Part model, mm, in its own coordinate system. Face numbers are marked on the shaded views. A direction names the side the tool comes from. Give positions to 0.01 mm unless a question says otherwise; leave off trailing zeros. Write each loop counter-clockwise with the first axis right and the second up, starting at its lowest first coordinate (ties: lowest second). Pieces come first, ordered by that corner, then holes. Notation, with made-up numbers: (-33, 85) - (-20, 85) arc R28 cw to (-20, 104) - close; hole circle Ø9 at (34, -39.75). An arc over 180 degrees is marked (long way). Answer as a JSON object with one key per item and string values. Group by question number.
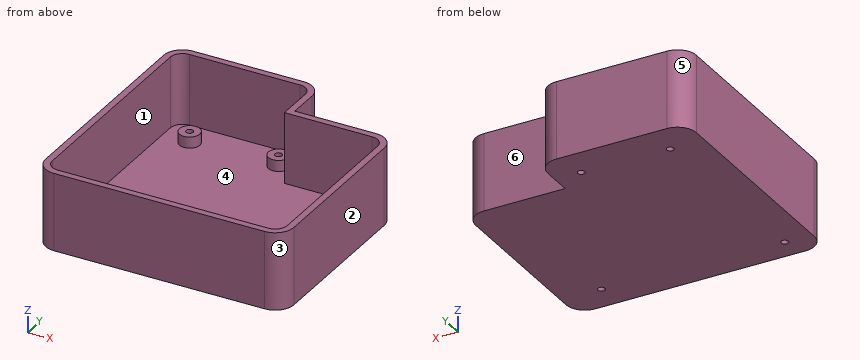
```python
from build123d import *

# Parameters (mm, degrees)
SKETCH1_R           = 1.6
BOSS_EXTRUDE1_DEPTH = 35
SHELL3_T            = -3
CUT_EXTRUDE2_DEPTH  = 27


with BuildPart() as part:
    # Sketch1 → Boss-Extrude1 (new body)
    with BuildSketch(Plane.XY):
        with BuildLine():
            Line((41.47958643, 169.703196001), (-8.43041357, 169.703196001))
            ThreePointArc((-8.43041357, 169.703196001), (-14.44082121, 167.213603641), (-16.93041357, 161.203196001))
            Line((-16.93041357, 161.203196001), (-16.93041357, 66.203196001))
            ThreePointArc((-16.93041357, 66.203196001), (-14.44082121, 60.192788361), (-8.43041357, 57.703196001))
            Line((-8.43041357, 57.703196001), (86.56958643, 57.703196001))
            ThreePointArc((86.56958643, 57.703196001), (92.57999407, 60.192788361), (95.06958643, 66.203196001))
            Line((95.06958643, 66.203196001), (95.06958643, 138.923196001))
            ThreePointArc((95.06958643, 138.923196001), (92.57999407, 144.933603641), (86.56958643, 147.423196001))
            Line((86.56958643, 147.423196001), (84.57958643, 147.423196001))
            Line((84.57958643, 147.423196001), (78.22958643, 147.423196001))
            Line((78.22958643, 147.423196001), (56.63958643, 147.423196001))
            Line((56.63958643, 147.423196001), (50.28958643, 147.423196001))
            Line((50.28958643, 147.423196001), (49.947630422, 147.423196001))
            Line((49.947630422, 147.423196001), (49.97958643, 161.203196001))
            ThreePointArc((49.97958643, 161.203196001), (47.48999407, 167.213603641), (41.47958643, 169.703196001))
        make_face()
        with Locations((-1.583516975, 154.760976138)):
            Circle(SKETCH1_R, mode=Mode.SUBTRACT)
        with Locations((38.108590224, 155.552573365)):
            Circle(SKETCH1_R, mode=Mode.SUBTRACT)
        with Locations((-4.549842033, 67.784537285)):
            Circle(SKETCH1_R, mode=Mode.SUBTRACT)
        with Locations((76.81802316, 70.207451643)):
            Circle(SKETCH1_R, mode=Mode.SUBTRACT)
    extrude(amount=BOSS_EXTRUDE1_DEPTH)

    # Shell3
    shell3_openings = [part.faces().sort_by_distance(p)[0] for p in [
        (36.150005596, 109.720855489, 35),
    ]]
    offset(amount=SHELL3_T, openings=shell3_openings, kind=Kind.INTERSECTION)

    # Sketch4 → Cut-Extrude2 (cut)
    with BuildSketch(Plane.XY.offset(35)):
        with BuildLine():
            Line((41.47958643, 164.703196001), (-8.43041357, 164.703196001))
            ThreePointArc((-8.43041357, 164.703196001), (-10.905287304, 163.678069735), (-11.93041357, 161.203196001))
            Line((-11.93041357, 161.203196001), (-11.93041357, 66.203196001))
            ThreePointArc((-11.93041357, 66.203196001), (-10.905287304, 63.728322267), (-8.43041357, 62.703196001))
            Line((-8.43041357, 62.703196001), (86.56958643, 62.703196001))
            ThreePointArc((86.56958643, 62.703196001), (89.044460164, 63.728322267), (90.06958643, 66.203196001))
            Line((90.06958643, 66.203196001), (90.06958643, 138.923196001))
            ThreePointArc((90.06958643, 138.923196001), (89.044460164, 141.398069735), (86.56958643, 142.423196001))
            Line((86.56958643, 142.423196001), (44.936021909, 142.423196001))
            Line((44.936021909, 142.423196001), (44.979583495, 161.207728174))
            ThreePointArc((44.979583495, 161.207728174), (43.95285728, 163.679671582), (41.47958643, 164.703196001))
        make_face()
    extrude(amount=-CUT_EXTRUDE2_DEPTH, mode=Mode.SUBTRACT)


solid = part.part
```
1) Saw through at D-D (x = 1.5). List the corners of the cut face in (y, z), and give its area (3 significant figures).
2) Saw through at A-A (z = 28). List the corners of the cut face in (x, y), and give its area (3 significant figures).
3) Two-plate mould, pull along Y, no slides. Class the marked faces 1, 2 and 3: +Y half, -Y half, draft (parallel to the pull), parting line (faces both ways), or undercut.
4) Drill centre lines: line 1 along X through (y, z) = (95.5, 17); line 2 along Y through (x, z) = (27.5, 14.5); line 3 along X through (y, z) = (161.5, 7). Where is each one in solid material? Low to high. Write a range as from..to.
5) Drop flat-ended pins along their axis: P1, Ø10, axis at x = -2, y = 156, coming from the +Z side; P2, Ø1.9, axis at x = -1.58, y = 154.76, coming from the +Z side; P3, Ø10.5, axis at x = 60.5, z = 23, coming from the +Y side. Give the stop position or say it passes through.
6) Saw through at C-C (x = 13). List the corners of the cut face in (y, z), and give its area (3 significant figures).
7) Which spindle directions (+Z, -Z, +X, -X, +Y, -Y) get a long thin tool onto all of the face, cutting with end or side? Do the marked faces 4, 5 and 6. Say none if no direction does.
8) Saw through at B-B (y = 81.5). List the corners of the cut face in (x, z), and give its area (3 significant figures).
Checks:
{
 "1": {"outline": "(57.7, 0) - (169.7, 0) - (169.7, 35) - (166.7, 35) - (166.7, 3) - (158.17, 3) - (158.17, 8) - (151.35, 8) - (151.35, 3) - (60.7, 3) - (60.7, 35) - (57.7, 35) - close", "area": "562 mm2"},
 "2": {"outline": "(-16.93, 66.2) arc R8.5 ccw to (-8.43, 57.7) - (86.57, 57.7) arc R8.5 ccw to (95.07, 66.2) - (95.07, 138.92) arc R8.5 ccw to (86.57, 147.42) - (49.95, 147.42) - (49.98, 161.2) arc R8.5 ccw to (41.48, 169.7) - (-8.43, 169.7) arc R8.5 ccw to (-16.93, 161.2) - close; hole (-13.93, 66.2) arc R5.5 ccw to (-8.43, 60.7) - (86.57, 60.7) arc R5.5 ccw to (92.07, 66.2) - (92.07, 138.92) arc R5.5 ccw to (86.57, 144.42) - (46.94, 144.42) - (46.98, 161.21) arc R5.5 ccw to (41.48, 166.7) - (-8.43, 166.7) arc R5.5 ccw to (-13.93, 161.2) - close", "area": "1,260 mm2"},
 "3": {"face 1": "undercut", "face 2": "draft", "face 3": "-Y half"},
 "4": {"line 1": "-16.93..-13.93, 92.07..95.07", "line 2": "57.7..60.7, 166.7..169.7", "line 3": "-16.93..-13.92, 46.97..49.97"},
 "5": {"P1": "z = 8", "P2": "through", "P3": "y = 147.42"},
 "6": {"outline": "(57.7, 0) - (169.7, 0) - (169.7, 35) - (166.7, 35) - (166.7, 3) - (60.7, 3) - (60.7, 35) - (57.7, 35) - close", "area": "528 mm2"},
 "7": {"face 4": "+Z", "face 5": "+Z, -Z, -X, +Y", "face 6": "+Z, -Z, +X, +Y"},
 "8": {"outline": "(-16.93, 0) - (95.07, 0) - (95.07, 35) - (92.07, 35) - (92.07, 3) - (-13.93, 3) - (-13.93, 35) - (-16.93, 35) - close", "area": "528 mm2"}
}
